```python
from build123d import *

# Parameters (mm, degrees)
SKETCH1_W           = 40
SKETCH1_H           = 100
BOSS_EXTRUDE2_DEPTH = 40
SKETCH2_R           = 14.3
CUT_EXTRUDE1_DEPTH  = 41
SKETCH3_W           = 34
SKETCH3_H           = 34
CUT_EXTRUDE2_DEPTH  = 101


with BuildPart() as part:
    # Sketch1 → Boss-Extrude2 (new body)
    with BuildSketch(Plane.XY):
        Rectangle(SKETCH1_W, SKETCH1_H)
    extrude(amount=BOSS_EXTRUDE2_DEPTH)

    # Sketch2 → Cut-Extrude1 (cut, through all)
    with BuildSketch(Plane.XY.offset(40)):
        with Locations((0, 28)):
            Circle(SKETCH2_R)
    extrude(amount=-CUT_EXTRUDE1_DEPTH, mode=Mode.SUBTRACT)

    # Sketch3 → Cut-Extrude2 (cut, through all)
    with BuildSketch(Plane(origin=(0, 50, 0), x_dir=(1, 0, 0), z_dir=(0, 1, 0))):
        with Locations((0, -20)):
            Rectangle(SKETCH3_W, SKETCH3_H)
    extrude(amount=-CUT_EXTRUDE2_DEPTH, mode=Mode.SUBTRACT)


solid = part.part
```
Check sheet for the modelled part. Datum: model origin and axes. Units: mm. A direction names the side the tool comes from. Coordinates: 2 decimals unless noted, no trailing zeros. Loops run counter-clockwise (first coordinate to the right, second up) from the corner with the lowest first, then second, coordinate; pieces in that order, holes last.
1) Sectioned sample at A-A (y = -32). Record the boundary of the cut face in (x, z), and give its area (3 significant figures).
2) Sectioned sample at B-B (z = 35.5). Record the boundary of the cut face in (x, y).
3) Release check for a two-part mould opening along X. For faces 1 (the face through (17, 1, 20)), 2 (the face through (0, 1, 0)), 3 (the face through (-20, -1, 20)) record: released by +X, released by -X, zero draft, split by the parting line, or undercut.
4) Sectioned sample at C-C (x = 0). Record the boundary of the cut face in (y, z).
5) Access from +Z, -Z, +X, -X, +Y, -Y to the whole of each face (thin tool, end or side, straight path). Record for faces 4 (the face through (-0.3, -50, 37.5)), 5 (the face through (0, -10, 37)).
6) Sectioned sample at D-D (y = 28). Record the boundary of the cut face in (x, z), and give its area (3 significant figures).
7) Material ranges on probe 1 along X at (y, z) = (-41.5, 7.5); probe 2 along Z at (x, y) = (8.5, 14.5); probe 3 along Y at (x, z) = (0, 38.1), recorded low to high.
8) Gauge pin test, flat end, axial feed: pin 1 (17 mm diameter, centred on x = 0, y = 28, fed in from +Z). Record the tip position at first contact, or that the pin passes through.
Check sheet entries:
1. outline: (-20, 0) - (20, 0) - (20, 40) - (-20, 40) - close; hole (-17, 3) - (17, 3) - (17, 37) - (-17, 37) - close
1. area: 444 mm2
2. outline: (-20, -50) - (-17, -50) - (-17, 50) - (-20, 50) - close; (17, -50) - (20, -50) - (20, 50) - (17, 50) - close
3. face 1: undercut
3. face 2: zero draft
3. face 3: released by -X
4. outline: (-50, 0) - (13.7, 0) - (13.7, 3) - (-50, 3) - close; (-50, 37) - (13.7, 37) - (13.7, 40) - (-50, 40) - close; (42.3, 0) - (50, 0) - (50, 3) - (42.3, 3) - close; (42.3, 37) - (50, 37) - (50, 40) - (42.3, 40) - close
5. face 4: +Z, -Z, +X, -X, -Y
5. face 5: +Y, -Y
6. outline: (-20, 0) - (-14.3, 0) - (-14.3, 3) - (-17, 3) - (-17, 37) - (-14.3, 37) - (-14.3, 40) - (-20, 40) - close; (14.3, 0) - (20, 0) - (20, 40) - (14.3, 40) - (14.3, 37) - (17, 37) - (17, 3) - (14.3, 3) - close
6. area: 272 mm2
7. probe 1: x = -20 to -17, 17 to 20
7. probe 2: z = 0 to 3, 37 to 40
7. probe 3: y = -50 to 13.7, 42.3 to 50
8. pin 1: passes through
